```python
from build123d import *

# Parameters (mm, degrees)
BOSS_EXTRUDE1_DEPTH = 15
SKETCH3_R           = 4.5
CUT_EXTRUDE1_DEPTH  = 110.607127014
SKETCH4_R           = 4.5
CUT_EXTRUDE2_DEPTH  = 95.229658783


with BuildPart() as part:
    # Sketch2 → Boss-Extrude1 (new body)
    with BuildSketch(Plane.XY):
        Polygon((-216.019091895, 17.382825188), (-212.930081555, 3.727862166), (-213.764027452, -4.398444723), (-213.764027452, -18.398444723), (-203.764027452, -18.398444723), (-203.764027452, -4.398444723), (-181.136073294, 5.936039038), (-176.194518086, -1.729112182), (-176.194518086, -18.398444723), (-166.194518086, -18.398444723), (-166.194518086, -6.398444723), (-150.828445352, 10.518587471), (-136.720595227, -6.398444723), (-136.720595227, -18.398444723), (-126.720595227, -18.398444723), (-126.720595227, -6.398444723), (-144.655266447, 19.172913865), (-147.744276787, 32.827876887), (-157.497821802, 30.62144093), (-154.408811463, 16.966477908), (-169.201460721, 2.373183741), (-173.915901493, 12.553605994), (-177.004911833, 26.208569016), (-186.758456849, 24.002133059), (-183.669446509, 10.347170037), (-202.433997642, 1.777153163), (-202.369507285, 2.366827181), (-206.265546879, 19.589261145), align=None)
    extrude(amount=BOSS_EXTRUDE1_DEPTH)

    # Sketch3 → Cut-Extrude1 (cut, through all)
    with BuildSketch(Plane(origin=(-201.761622141, -45.642286691, 0), x_dir=(0, 0, 1), z_dir=(-0.9753545015403321, -0.22064359570359257, 0))):
        with Locations(Location((7.5, 56.617645973, 0), (0, 0, 270))):
            Circle(SKETCH3_R)
        with BuildLine():
            Line((15, 59.617645973), (20.879218682, 59.617645973))
            Line((20.879218682, 59.617645973), (20.879218682, 67.791125086))
            Line((20.879218682, 67.791125086), (14.372574649, 67.791125086))
            Line((14.372574649, 67.791125086), (-2.562016451, 67.791125086))
            Line((-2.562016451, 67.791125086), (-2.562016451, 59.617645973))
            Line((-2.562016451, 59.617645973), (0, 59.617645973))
            ThreePointArc((0, 59.617645973), (1.464466094, 63.153179879), (5, 64.617645973))
            Line((5, 64.617645973), (8.859819986, 64.617645973))
            Line((8.859819986, 64.617645973), (10, 64.617645973))
            ThreePointArc((10, 64.617645973), (13.535533906, 63.153179879), (15, 59.617645973))
        make_face()
    extrude(amount=-CUT_EXTRUDE1_DEPTH, mode=Mode.SUBTRACT)

    # Sketch4 → Cut-Extrude2 (cut, through all)
    with BuildSketch(Plane.ZY.offset(213.764027452)):
        with Locations(Location((7.5, -10.398444723, 0), (0, 0, 62.733955549))):
            Circle(SKETCH4_R)
        with BuildLine():
            Line((5, -18.398444723), (10, -18.398444723))
            ThreePointArc((10, -18.398444723), (13.535533906, -16.933978629), (15, -13.398444723))
            Line((15, -13.398444723), (20.19317818, -13.398444723))
            Line((20.19317818, -13.398444723), (20.19317818, -22.025318281))
            Line((20.19317818, -22.025318281), (-2.656583896, -22.025318281))
            Line((-2.656583896, -22.025318281), (-2.656583896, -13.398444723))
            Line((-2.656583896, -13.398444723), (0, -13.398444723))
            ThreePointArc((0, -13.398444723), (1.464466094, -16.933978629), (5, -18.398444723))
        make_face()
    extrude(amount=-CUT_EXTRUDE2_DEPTH, mode=Mode.SUBTRACT)


solid = part.part
```
Verification items for the finished model (mm, model axes). A direction names the side the tool comes from. Coordinates: 2 decimals unless noted, no trailing zeros. Write each loop counter-clockwise with the first axis right and the second up, starting at its lowest first coordinate (ties: lowest second). Pieces come first, ordered by that corner, then holes. Notation, with made-up numbers: (23, 69) - (44, 69) arc R19 cw to (44, 102) - close; hole circle Ø9 at (18.25, -33). An arc over 180 degrees is marked (long way). Write item = value, one per line.
Q1. Cross-section at B-B (z = 13). Enter the section's corners in (x, y), plus the area to 3 significant figures.
Answer:
outline = (-215.8, 16.41) - (-212.93, 3.73) - (-213.76, -4.4) - (-213.76, -17.4) - (-203.76, -17.4) - (-203.76, -4.4) - (-181.14, 5.94) - (-176.19, -1.73) - (-176.19, -17.4) - (-166.19, -17.4) - (-166.19, -6.4) - (-150.83, 10.52) - (-136.72, -6.4) - (-136.72, -17.4) - (-126.72, -17.4) - (-126.72, -6.4) - (-144.66, 19.17) - (-147.52, 31.85) - (-157.28, 29.65) - (-154.41, 16.97) - (-169.2, 2.37) - (-173.92, 12.55) - (-176.78, 25.23) - (-186.54, 23.03) - (-183.67, 10.35) - (-202.43, 1.78) - (-202.37, 2.37) - (-206.04, 18.61) - close
area = 1,570 mm²
Q2. Cross-section at C-C (x = -208). Give the number of separate pieces and of enclosed holes in the cut face, plus the area to 3 significant figures.
Answer:
separate_pieces = 1
enclosed_holes = 2
area = 413 mm²
Q3. Mould release check, pull along X, two halves, no side actions. Record for faces 1 (the face through (-208.83, -16.97, 13.5)), 2 (the face through (-213.34, -0.28, 7.4)), 3 (the face through (-156.66, 26.92, 10.73)): released by +X, released by -X, zero draft, split by the parting line, or undercut.
Answer:
face_1 = zero draft
face_2 = released by -X
face_3 = undercut
Q4. Material ranges on L1, parallel to X at y = -15.5, z = 3.25; L2, parallel to X at y = -1, z = 4; L3, parallel to X at y = 7.5, z = 3.25, recorded low to high. Write a range as from..to.
Answer:
L1 = -213.76..-203.76, -176.19..-166.19, -136.72..-126.72
L2 = -213.42..-196.32, -176.66..-161.29, -141.22..-130.51
L3 = -213.78..-203.53, -189.9..-171.58, -164..-153.57, -148.31..-136.47
Q5. Access from +Z, -Z, +X, -X, +Y, -Y to the whole of each face (thin tool, end or side, straight path). Record for faces 4 (the face through (-161.702, 9.772, 7.395)), 5 (the face through (-203.764, -15, 6)), 6 (the face through (-171.265, -16.895, 1.426)).
Answer:
face_4 = +Z, -Z
face_5 = +Z, -Z, -Y
face_6 = -Z, +X, -X, -Y
Q6. Go/stop test with flat-tipped pins: pin 1 Ø2 at (y, z) = (24.5, 1.5) entering from +X; pin 2 Ø4.5 at (y, z) = (-13.5, 6) entering from -X; pin 3 Ø6 at (y, z) = (-12, 4) entering from +X; pin 4 Ø3 at (x, z) = (-149.5, 13) entering from -Y. Record where each tip stops, or that it passes through.
Answer:
pin_1 = -145.63
pin_2 = -213.76
pin_3 = -126.72
pin_4 = 7.13
Q7. Cross-section at A-A (y = -10). Enter the section's corners in (x, z).
Answer:
outline = (-213.76, 0) - (-203.76, 0) - (-203.76, 3.02) - (-213.76, 3.02) - close; (-213.76, 11.98) - (-203.76, 11.98) - (-203.76, 15) - (-213.76, 15) - close; (-176.19, 0) - (-166.19, 0) - (-166.19, 3.02) - (-176.19, 3.02) - close; (-176.19, 11.98) - (-166.19, 11.98) - (-166.19, 15) - (-176.19, 15) - close; (-136.72, 0) - (-126.72, 0) - (-126.72, 3.02) - (-136.72, 3.02) - close; (-136.72, 11.98) - (-126.72, 11.98) - (-126.72, 15) - (-136.72, 15) - close
